Geometry check sheet. Reference: the model listing, model coordinates, mm. Face numbers are marked on the shaded views. A direction names the side the tool comes from. Round coordinates to 2 decimals unless told otherwise and drop trailing zeros. Order: outer loops, then holes, each group sorted by start corner. A loop starts at its lowest first (then second) coordinate and runs counter-clockwise, first axis right, second up.
```python
from build123d import *

# Parameters (mm, degrees)
F1_DEPTH = 3
F2_R     = 6.5
F3_DEPTH = 115
F4_W     = 28.374873
F4_H     = 45.940291
F5_DEPTH = 25
F6_DEPTH = 25


with BuildPart() as f1:
    # F0 (on Front) → F1 (new body)
    with BuildSketch(Plane.XZ):
        Polygon((0, 115), (0, 0), (48, 0), (48, 34.5), (35, 34.5), (35, 80.5), (48, 80.5), (48, 115), align=None)
    extrude(amount=F1_DEPTH)

    # F2 (on Top) → F3 (join)
    with BuildSketch(Plane.XY):
        with Locations((48.124816, -6.420063)):
            Circle(F2_R)
    extrude(amount=F3_DEPTH)

    # F4 (on Front) → F5 (cut)
    with BuildSketch(Plane.XZ):
        with Locations((51.307272, 57.549083)):
            Rectangle(F4_W, F4_H)
    extrude(amount=F5_DEPTH, mode=Mode.SUBTRACT)

    # F4 (on Front) → F6 (cut)
    with BuildSketch(Plane.XZ):
        with Locations((51.307272, 57.549083)):
            Rectangle(F4_W, F4_H)
    extrude(amount=-F6_DEPTH, mode=Mode.SUBTRACT)


solid = f1.part
```
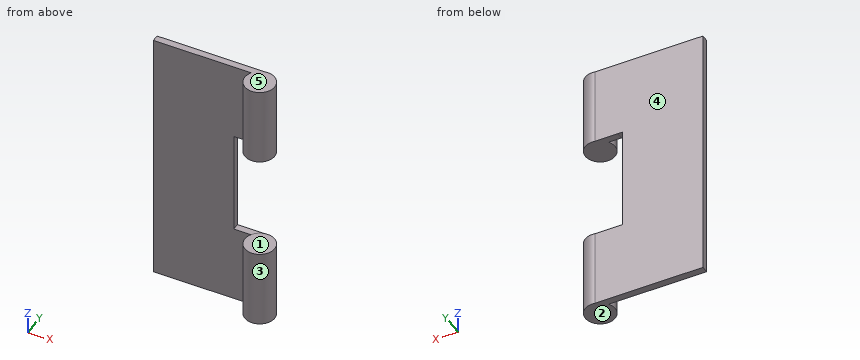
(1) Sectioned sample at C-C, the plane z = 22.5. Record the cut outline in (x, y), and give its area (3 significant figures).
Returned:
outline: (0, -3) - (42.6, -3) arc R6.5 ccw (long way) to (47.11, 0) - (0, 0) - close
area: 265 mm2
(2) Sectioned sample at D-D, the plane x = 32. Record the cut outline in (y, z), and give its area (3 significant figures).
Returned:
outline: (-3, 0) - (0, 0) - (0, 115) - (-3, 115) - close
area: 345 mm2
(3) Sectioned sample at A-A, the plane x = 39. Record the cut outline in (y, z), and give its area (3 significant figures).
Returned:
outline: (-3, 0) - (0, 0) - (0, 34.5) - (-3, 34.5) - close; (-3, 80.52) - (0, 80.52) - (0, 115) - (-3, 115) - close
area: 207 mm2
(4) Material ranges on line 1 (Z direction, x = 43, y = -3); line 2 (X direction, y = -6, z = 86.5); line 3 (Y direction, x = 22, z = 98.5), recorded low to high.
Returned:
line 1: z = 0 to 34.58, 80.52 to 115
line 2: x = 41.64 to 54.61
line 3: y = -3 to 0
(5) Draft check along Y on the marked faces 3, 4 and 5. Enter one of: released by +Y, released by -Y, zero draft, split by the parting line, or undercut.
Returned:
face 3: undercut
face 4: released by +Y
face 5: zero draft
(6) Set-up check for the marked faces 1 and 2: record each of +Z, -Z, +X, -X, +Y, -Y from which the full face is reachable in a straight line by a thin tool's end or side.
Returned:
face 1: +X, +Y, -Y
face 2: -Z, +X, -X, +Y, -Y
(7) Sectioned sample at B-B, the plane y = -4.5. Record the cut outline in (x, z), and give its area (3 significant figures).
Returned:
outline: (41.91, 0) - (54.33, 0) - (54.33, 34.58) - (41.91, 34.58) - close; (41.91, 80.52) - (54.33, 80.52) - (54.33, 115) - (41.91, 115) - close
area: 858 mm2
(8) Depth check by flat-ended pin: P1, Ø1, axis at y = -9.5, z = 90.5, coming from the +X side; P2, Ø14, axis at x = 13.5, z = 86, coming from the +Y side; P3, Ø1.5, axis at y = -5, z = 31.5, coming from the -X side. Enter the tip coordinate at first touch or a pass-through.
Returned:
P1: stops at x = 54.09
P2: stops at y = 0
P3: stops at x = 41.66
